Autodesk Inventor part; units mm, degrees
ref_plane "YZ Plane" through (0, 0, 0) normal (1, 0, 0) x (0, 1, 0)
ref_plane "XZ Plane" through (0, 0, 0) normal (0, 1, 0) x (-1, 0, 0)
ref_plane "XY Plane" through (0, 0, 0) normal (0, 0, 1) x (1, 0, 0)
sketch "Sketch1" plane through (0, 0, 0) normal (0, 1, 0) x (-1, 0, 0)
  line L0 (-25, 175) -> (25, 175)
  line L1 (25, 175) -> (25, -175)
  line L2 (25, -175) -> (-25, -175)
  line L3 (-25, -175) -> (-25, 175)
  line L4 (-25, 175) -> (25, -175) construction
  line L5 (25, 175) -> (-25, -175) construction
  line L6 (0, 175) -> (0, 165)
  circle A0 centre (0, 165) radius 4
  line L7 (0, 165) -> (0, 115)
  circle A1 centre (0, 115) radius 4
  point P0 (0, 0)
  dimension "d0" = 50
  dimension "d1" = 350
  dimension "d2" = 10
  dimension "d3" = 8
  dimension "d4" = 50
  dimension "d5" = 8
extrude "Extrusion1" add sketch "Sketch1" along normal blind 2
properties part number "Ldw"
Verification items for the finished model (mm, model axes). Give positions to 0.01 mm unless a question says otherwise; leave off trailing zeros. Loops run counter-clockwise (first coordinate to the right, second up) from the corner with the lowest first, then second, coordinate; pieces in that order, holes last.
1. Section check A-A, the plane z = 165. Enter the section's corners in (x, y).
2. Section check B-B, the plane x = 0. Enter the section's corners in (y, z), then the cut area to 3 significant figures.
3. Thickness scan on line 1 (Z direction, x = 0, y = 1.45); line 2 (X direction, y = 1.4, z = 165). Record the ranges inside material, lowest first.
4. Mould release check, pull along X, two halves, no side actions. Record for faces 1 (the cylindrical face through (0.521, 0.986, 111.034)), 2 (the flat face through (0, 0, 2)): released by +X, released by -X, zero draft, split by the parting line, or undercut.
Geometry says:
1. outline: (-25, 0) - (-4, 0) - (-4, 2) - (-25, 2) - close; (4, 0) - (25, 0) - (25, 2) - (4, 2) - close
2. outline: (0, -175) - (2, -175) - (2, 111) - (0, 111) - close; (0, 119) - (2, 119) - (2, 161) - (0, 161) - close; (0, 169) - (2, 169) - (2, 175) - (0, 175) - close
2. area: 668 mm2
3. line 1: z = -175 to 111, 119 to 161, 169 to 175
3. line 2: x = -25 to -4, 4 to 25
4. face 1: undercut
4. face 2: zero draft
